from build123d import *

# Parameters (mm, degrees)
SKETCH1_R           = 24.66826923
SKETCH1_R_2         = 1.8669
BOSS_EXTRUDE1_DEPTH = 2.79
SKETCH2_R           = 20.865
SKETCH2_R_2         = 4.465
CUT_EXTRUDE1_DEPTH  = 1.3
SKETCH3_R           = 4.445
CUT_EXTRUDE2_DEPTH  = 36.147765414


with BuildPart() as part:
    # Sketch1 → Boss-Extrude1 (new, symmetric)
    with BuildSketch(Plane.XY):
        Circle(SKETCH1_R)
        Circle(SKETCH1_R_2, mode=Mode.SUBTRACT)
    extrude(amount=BOSS_EXTRUDE1_DEPTH, both=True)

    # Sketch2 → Cut-Extrude1 (cut)
    with BuildSketch(Plane.XY.offset(2.79)):
        Circle(SKETCH2_R)
        Circle(SKETCH2_R_2, mode=Mode.SUBTRACT)
    cut_extrude1 = extrude(amount=-CUT_EXTRUDE1_DEPTH, mode=Mode.SUBTRACT)

    # Sketch3 → Cut-Extrude2 (cut, through all)
    with BuildSketch(Plane.XY.offset(1.49)):
        with Locations((0, 9.9568)):
            Circle(SKETCH3_R)
        with Locations((9.9568, 0)):
            Circle(SKETCH3_R)
        with Locations((0, -9.9568)):
            Circle(SKETCH3_R)
        with Locations((-9.9568, 0)):
            Circle(SKETCH3_R)
    extrude(amount=-CUT_EXTRUDE2_DEPTH, mode=Mode.SUBTRACT)

    # Mirror1: Cut-Extrude1 across plane
    add(cut_extrude1.mirror(Plane.XY), mode=Mode.SUBTRACT)


solid = part.part
Input: part model. Units: mm. Frame: model coordinates. A direction names the side the tool comes from. Give positions to 0.01 mm unless a question says otherwise; leave off trailing zeros. Write each loop counter-clockwise with the first axis right and the second up, starting at its lowest first coordinate (ties: lowest second). Pieces come first, ordered by that corner, then holes.
Q1. Section A-A, the plane z = -2.1. Output: boundary loops of the cut face in (x, y) (3 decimals), plus the area to 3 significant figures.
Q2. Set-up query: faces 1 (the face through (0, 5, -1.49)), 2 (the face through (-14.398, 0.195, 0.021)), 3 (the face through (0, 5, 1.49)). Return all of +Z, -Z, +X, -X, +Y, -Y with unobstructed straight access to the full face (end or side cutting, diameter ignored); none if empty.
Q3. Section B-B, the plane y = 0. State how many separate pieces and enclosed holes the cut face has, plus the area to 3 significant figures.
Q4. First-contact query: P1, Ø5, axis at x = 14, y = -10, coming from the -Z side; P2, Ø3, axis at x = 5.5, z = -2, coming from the +Y side. Flat tips, straight axial feed; report the tip coordinate or a pass-through.
Q5. Pull-direction query (X, two-part tool) for faces 4 (the face through (-18, 11, 2.79)), 5 (the face through (-0.964, 5.618, 0.021)), 6 (the face through (13.26, 20.8, 0.04)); classes: pulls with the +X half, pulls with the -X half, needs draft (parallel to the pull), parting line crosses it, or undercut.
Q6. Material intervals for probe 1 along Y at (x, z) = (0.5, -2); probe 2 along X at (y, z) = (2.5, -1.45); probe 3 along Y at (x, z) = (-0.5, -0.65), sorted ascending.
Q7. Section D-D, the plane y = 7. Output: boundary loops of the cut face in (x, z), plus the area to 3 significant figures.
Filled in:
1. outline: circle Ø49.337 at (0, 0); circle Ø8.93 at (0, 0); hole circle Ø41.73 at (0, 0); hole circle Ø3.734 at (0, 0)
1. area: 596 mm2
2. face 1: -Z
2. face 2: +Z, -Z
2. face 3: +Z
3. separate pieces: 4
3. enclosed holes: 0
3. area: 116 mm2
4. P1: stops at z = -1.49
4. P2: stops at y = 24.34
5. face 4: needs draft
5. face 5: undercut
5. face 6: parting line crosses it
6. probe 1: y = -24.66 to -20.86, -4.44 to -1.8, 1.8 to 4.44, 20.86 to 24.66
6. probe 2: x = -24.54 to -13.63, -6.28 to 6.28, 13.63 to 24.54
6. probe 3: y = -24.66 to -14.37, -5.54 to -1.8, 1.8 to 5.54, 14.37 to 24.66
7. outline: (-23.65, -2.79) - (-19.66, -2.79) - (-19.66, -1.49) - (-3.32, -1.49) - (-3.32, 1.49) - (-19.66, 1.49) - (-19.66, 2.79) - (-23.65, 2.79) - close; (3.32, -1.49) - (19.66, -1.49) - (19.66, -2.79) - (23.65, -2.79) - (23.65, 2.79) - (19.66, 2.79) - (19.66, 1.49) - (3.32, 1.49) - close
7. area: 142 mm2
